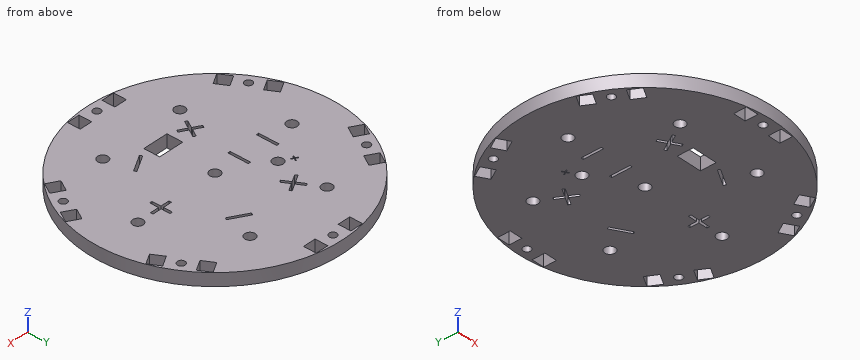
```python
from build123d import *

# Parameters (mm, degrees)
BOSS_EXTRU_1_OUTLINE_R   = 50
BOSS_EXTRU_1_OUTLINE_W   = 5
BOSS_EXTRU_1_OUTLINE_H   = 5
BOSS_EXTRU_1_OUTLINE_R_2 = 2.05
BOSS_EXTRU_1_OUTLINE_R_3 = 1.5
BOSS_EXTRU_1_DEPTH       = 5
SKETCH3_W                = 1
SKETCH3_H                = 8
SKETCH3_W_2              = 10
SKETCH3_H_2              = 6.223903135
CUT_EXTRUDE2_DEPTH       = 10


# Read off the part's stored shape, not the designer's step: Boss.-Extru.1
with BuildPart() as part:
    # Boss.-Extru.1 outline → Boss.-Extru.1 (new body)
    with BuildSketch(Plane.XY):
        Circle(BOSS_EXTRU_1_OUTLINE_R)
        Polygon((-37.262039705, -33.060254038), (-39.762039705, -28.730127019), (-35.431912686, -26.230127019), (-32.931912686, -30.560254038), align=None, mode=Mode.SUBTRACT)
        with Locations((-7.5, -46.3)):
            Rectangle(BOSS_EXTRU_1_OUTLINE_W, BOSS_EXTRU_1_OUTLINE_H, mode=Mode.SUBTRACT)
        with Locations((-16.666666667, -28.867513459)):
            Circle(BOSS_EXTRU_1_OUTLINE_R_2, mode=Mode.SUBTRACT)
        with Locations((-40.096976195, -23.15)):
            Circle(BOSS_EXTRU_1_OUTLINE_R_3, mode=Mode.SUBTRACT)
        Polygon((-42.931912686, -13.239745962), (-40.431912686, -17.569872981), (-44.762039705, -20.069872981), (-47.262039705, -15.739745962), align=None, mode=Mode.SUBTRACT)
        with Locations((0, -46.3)):
            Circle(BOSS_EXTRU_1_OUTLINE_R_3, mode=Mode.SUBTRACT)
        with Locations((7.5, -46.3)):
            Rectangle(BOSS_EXTRU_1_OUTLINE_W, BOSS_EXTRU_1_OUTLINE_H, mode=Mode.SUBTRACT)
        with Locations((16.666666667, -28.867513459)):
            Circle(BOSS_EXTRU_1_OUTLINE_R_2, mode=Mode.SUBTRACT)
        Polygon((32.931912686, -30.560254038), (35.431912686, -26.230127019), (39.762039705, -28.730127019), (37.262039705, -33.060254038), align=None, mode=Mode.SUBTRACT)
        with Locations((40.096976195, -23.15)):
            Circle(BOSS_EXTRU_1_OUTLINE_R_3, mode=Mode.SUBTRACT)
        Polygon((47.262039705, -15.739745962), (44.762039705, -20.069872981), (40.431912686, -17.569872981), (42.931912686, -13.239745962), align=None, mode=Mode.SUBTRACT)
        with Locations((-33.333333333, 0)):
            Circle(BOSS_EXTRU_1_OUTLINE_R_2, mode=Mode.SUBTRACT)
        Polygon((-47.262039705, 15.739745962), (-44.762039705, 20.069872981), (-40.431912686, 17.569872981), (-42.931912686, 13.239745962), align=None, mode=Mode.SUBTRACT)
        with Locations((-40.096976195, 23.15)):
            Circle(BOSS_EXTRU_1_OUTLINE_R_3, mode=Mode.SUBTRACT)
        with Locations((-16.671397032, 9.625235564)):
            Circle(BOSS_EXTRU_1_OUTLINE_R_2, mode=Mode.SUBTRACT)
        Polygon((-32.931912686, 30.560254038), (-35.431912686, 26.230127019), (-39.762039705, 28.730127019), (-37.262039705, 33.060254038), align=None, mode=Mode.SUBTRACT)
        with Locations((-16.666666667, 28.867513459)):
            Circle(BOSS_EXTRU_1_OUTLINE_R_2, mode=Mode.SUBTRACT)
        with Locations((-7.5, 46.3)):
            Rectangle(BOSS_EXTRU_1_OUTLINE_W, BOSS_EXTRU_1_OUTLINE_H, mode=Mode.SUBTRACT)
        Circle(BOSS_EXTRU_1_OUTLINE_R_2, mode=Mode.SUBTRACT)
        with Locations((33.333333333, 0)):
            Circle(BOSS_EXTRU_1_OUTLINE_R_2, mode=Mode.SUBTRACT)
        Polygon((42.931912686, 13.239745962), (40.431912686, 17.569872981), (44.762039705, 20.069872981), (47.262039705, 15.739745962), align=None, mode=Mode.SUBTRACT)
        with Locations((40.096976195, 23.15)):
            Circle(BOSS_EXTRU_1_OUTLINE_R_3, mode=Mode.SUBTRACT)
        with Locations((16.666666667, 28.867513459)):
            Circle(BOSS_EXTRU_1_OUTLINE_R_2, mode=Mode.SUBTRACT)
        with Locations((0, 46.3)):
            Circle(BOSS_EXTRU_1_OUTLINE_R_3, mode=Mode.SUBTRACT)
        with Locations((7.5, 46.3)):
            Rectangle(BOSS_EXTRU_1_OUTLINE_W, BOSS_EXTRU_1_OUTLINE_H, mode=Mode.SUBTRACT)
        Polygon((37.262039705, 33.060254038), (39.762039705, 28.730127019), (35.431912686, 26.230127019), (32.931912686, 30.560254038), align=None, mode=Mode.SUBTRACT)
    extrude(amount=BOSS_EXTRU_1_DEPTH)

    # Sketch3 → Cut-Extrude2 (cut)
    with BuildSketch(Plane.XY.offset(5)):
        with Locations((-10.5, 0)):
            Rectangle(SKETCH3_W, SKETCH3_H)
        with Locations((-22.833333333, 0)):
            Rectangle(SKETCH3_W, SKETCH3_H)
        Polygon((-13.233653965, 23.921361037), (-14.099679369, 23.421361037), (-12.349679369, 20.390272124), (-15.380768282, 18.640272124), (-14.880768282, 17.77424672), (-11.849679369, 19.52424672), (-10.099679369, 16.493157806), (-9.233653965, 16.993157806), (-10.983653965, 20.02424672), (-7.952565052, 21.77424672), (-8.452565052, 22.640272124), (-11.483653965, 20.890272124), align=None)
        Polygon((15.130768282, 18.207259422), (14.630768282, 17.341234018), (7.702565052, 21.341234018), (8.202565052, 22.207259422), align=None)
        Polygon((8.202565052, -22.207259422), (7.702565052, -21.341234018), (14.630768282, -17.341234018), (15.130768282, -18.207259422), align=None)
        Polygon((27.333333333, -0.5), (27.333333333, 0.5), (23.833333333, 0.5), (23.833333333, 4), (22.833333333, 4), (22.833333333, 0.5), (19.333333333, 0.5), (19.333333333, -0.5), (22.833333333, -0.5), (22.833333333, -4), (23.833333333, -4), (23.833333333, -0.5), align=None)
        Polygon((-14.099679369, -23.421361037), (-13.233653965, -23.921361037), (-11.483653965, -20.890272124), (-8.452565052, -22.640272124), (-7.952565052, -21.77424672), (-10.983653965, -20.02424672), (-9.233653965, -16.993157806), (-10.099679369, -16.493157806), (-11.849679369, -19.52424672), (-14.880768282, -17.77424672), (-15.380768282, -18.640272124), (-12.349679369, -20.390272124), align=None)
        with Locations((-0.211745945, -20.453185586)):
            Rectangle(SKETCH3_W_2, SKETCH3_H_2)
        Polygon((-20.834234776, 12.184801987), (-19.940304487, 11.668776346), (-20.102964744, 11.386925384), (-20.996895032, 11.902951025), (-21.517828526, 11.000607275), (-21.800380609, 11.163968654), (-21.279447115, 12.066312404), (-22.173377404, 12.582338045), (-22.010717147, 12.864189006), (-21.116786859, 12.348163365), (-20.596554487, 13.24840375), (-20.314002404, 13.085042371), align=None)
    extrude(amount=-CUT_EXTRUDE2_DEPTH, mode=Mode.SUBTRACT)


solid = part.part
```
The model under review builds one solid part; all positions refer to its coordinate system, in mm. Round coordinates to 2 decimals unless told otherwise and drop trailing zeros. Loops run counter-clockwise (first coordinate to the right, second up) from the corner with the lowest first, then second, coordinate; pieces in that order, holes last. Notation, with made-up numbers: (72.25, 49) -> (88.25, 49) arc R19 ccw to (88.25, 76) -> close; hole circle Ø10 at (-34, -28.5). An arc over 180 degrees is marked (long way). Answer as a JSON object with one key per item and string values. Group by question number.
1) We need section A-A on x = 0. Write out the cut boundary in (y, z).
2) For pin 1 Ø2.5 at (y, z) = (47, 3) entering from +X; pin 2 Ø2 at (x, z) = (-11, 4) entering from -Y; pin 3 Ø2.5 at (y, z) = (46, 1.5) entering from +X; pin 4 Ø1 at (x, y) = (34.5, 38) entering from -Z, all flat-tipped, find the tip position at first contact; note any pin that passes through.
3) We need section C-C on x = 30. Write out the cut boundary in (y, z).
4) For line 1 (Y direction, x = 0, z = 3.15); line 2 (Y direction, x = 39.5, z = 0.7); line 3 (X direction, y = 29, z = 3.45), list the stretches that pass through material, from the lowest coordinate up. Write a range as [from, to].
5) We need section B-B on y = 46.3. Write out the cut boundary in (x, z).
6) We need section D-D on z = 1.25. Give the number of separate pieces and of enclosed holes in the cut face, then the cut area to 3 significant figures.
Result set:
{
 "1": {"outline": "(-50, 0) -> (-47.8, 0) -> (-47.8, 5) -> (-50, 5) -> close; (-44.8, 0) -> (-23.57, 0) -> (-23.57, 5) -> (-44.8, 5) -> close; (-17.34, 0) -> (-2.05, 0) -> (-2.05, 5) -> (-17.34, 5) -> close; (2.05, 0) -> (44.8, 0) -> (44.8, 5) -> (2.05, 5) -> close; (47.8, 0) -> (50, 0) -> (50, 5) -> (47.8, 5) -> close"},
 "2": {"pin 1": "x = 20.17", "pin 2": "y = -48.99", "pin 3": "x = 22.3", "pin 4": "through"},
 "3": {"outline": "(-40, 0) -> (40, 0) -> (40, 5) -> (-40, 5) -> close"},
 "4": {"line 1": "[-50, -47.8], [-44.8, -23.57], [-17.34, -2.05], [2.05, 44.8], [47.8, 50]", "line 2": "[-30.66, -29.18], [-28.58, -24.53], [-21.77, 21.77], [24.53, 28.58], [29.18, 30.66]", "line 3": "[-40.73, -39.61], [-33.83, -18.71], [-14.62, 14.62], [18.71, 33.83], [39.61, 40.73]"},
 "5": {"outline": "(-18.88, 0) -> (-10, 0) -> (-10, 5) -> (-18.88, 5) -> close; (-5, 0) -> (-1.5, 0) -> (-1.5, 5) -> (-5, 5) -> close; (1.5, 0) -> (5, 0) -> (5, 5) -> (1.5, 5) -> close; (10, 0) -> (18.88, 0) -> (18.88, 5) -> (10, 5) -> close"},
 "6": {"separate pieces": "1", "enclosed holes": "35", "area": "7,270 mm²"}
}
